```python
from build123d import *

# Parameters (mm, degrees)
BOSS_EXTRUDE1_DEPTH     = 106
SKETCH3_R               = 5
BOSS_EXTRUDE2_DEPTH     = 61.5
BOSS_EXTRUDE3_START     = -25
BOSS_EXTRUDE3_DEPTH     = 70.666666667
BOSS_EXTRUDE4_DEPTH     = 2.5
FILLET2_R               = 10
CUT_EXTRUDE1_DEPTH      = 107
CUT_EXTRUDE1_DEPTH_BACK = 26
SKETCH7_R               = 20
SKETCH7_R_2             = 10
BOSS_EXTRUDE5_DEPTH     = 106
CUT_EXTRUDE2_DEPTH      = 1
CUT_EXTRUDE2_DEPTH_BACK = 132


with BuildPart() as part:
    # Sketch2 → Boss-Extrude1 (new body)
    with BuildSketch(Plane(origin=(0, 0, 0), x_dir=(1, 0, 0), z_dir=(0, 1, 0))):
        Polygon((0, -61.5), (0, 61.5), (-106, 0), align=None)
        Polygon((-10, 44.136889641), (-86.073338243, 0), (-10, -44.136889641), align=None, mode=Mode.SUBTRACT)
    extrude(amount=BOSS_EXTRUDE1_DEPTH)

    # Sketch3 → Boss-Extrude2 (add, symmetric)
    with BuildSketch(Plane.XY):
        with BuildLine():
            Line((0, 0), (50, 0))
            Line((50, 0), (91.711375741, 35))
            Line((91.711375741, 35), (150.654022129, 35))
            Line((150.654022129, 35), (201, -25))
            Line((201, -25), (246, -25))
            Line((246, -25), (246, -19))
            Line((246, -19), (246, -5))
            Line((246, -5), (231, -5))
            ThreePointArc((231, -5), (223.928932188, -7.928932188), (221, -15))
            Line((221, -15), (221, -19))
            Line((221, -19), (203.797845949, -19))
            Line((203.797845949, -19), (153.451868078, 41))
            Line((153.451868078, 41), (89.527554335, 41))
            Line((89.527554335, 41), (47.816178594, 6))
            Line((47.816178594, 6), (0, 6))
            Line((0, 6), (0, 0))
        make_face()
        with Locations((231, -15)):
            Circle(SKETCH3_R, mode=Mode.SUBTRACT)
    extrude(amount=BOSS_EXTRUDE2_DEPTH, both=True)

    # Sketch4 → Boss-Extrude3 (add)
    with BuildSketch(Plane(origin=(0, 0, 0), x_dir=(1, 0, 0), z_dir=(0, 1, 0)).offset(BOSS_EXTRUDE3_START)):
        Polygon((246, -30), (246, 30), (291, 0), align=None)
        Polygon((256, 11.314829082), (272.972243623, 0), (256, -11.314829082), align=None, mode=Mode.SUBTRACT)
    extrude(amount=BOSS_EXTRUDE3_DEPTH)

    # Sketch5 → Boss-Extrude4 (add, symmetric)
    with BuildSketch(Plane.XY):
        with BuildLine():
            Line((0, 106), (183.326730095, 106))
            Line((183.326730095, 106), (233.952407843, 45.666666667))
            Line((233.952407843, 45.666666667), (246, 45.666666667))
            Line((246, 45.666666667), (246, -5))
            Line((246, -5), (231, -5))
            ThreePointArc((231, -5), (223.928932188, -7.928932188), (221, -15))
            Line((221, -15), (221, -19))
            Line((221, -19), (203.797845949, -19))
            Line((203.797845949, -19), (153.451868078, 41))
            Line((153.451868078, 41), (89.527554335, 41))
            Line((89.527554335, 41), (47.816178594, 6))
            Line((47.816178594, 6), (0, 6))
            Line((0, 6), (0, 106))
        make_face()
    extrude(amount=BOSS_EXTRUDE4_DEPTH, both=True)

    # Fillet2
    fillet2_edges = [part.edges().sort_by_distance(p)[0] for p in [
        (50, 0, 0),
        (91.711375741, 35, 0),
        (150.654022129, 35, 0),
        (201, -25, 0),
        (203.797845949, -19, 32),
        (153.451868078, 41, 32),
        (89.527554335, 41, 32),
        (47.816178594, 6, 32),
        (47.816178594, 6, -32),
        (89.527554335, 41, -32),
        (153.451868078, 41, -32),
        (203.797845949, -19, -32),
        (233.952407843, 45.666666667, 0),
        (183.326730095, 106, 0),
    ]]
    fillet(fillet2_edges, radius=FILLET2_R)

    # Sketch6 → Cut-Extrude1 (cut, two sides)
    with BuildSketch(Plane(origin=(0, 0, 0), x_dir=(1, 0, 0), z_dir=(0, 1, 0))) as cut_extrude1_sk:
        Polygon((0, 61.5), (246, 61.5), (246, 30), align=None)
        Polygon((0, -61.5), (246, -30), (246, -61.5), align=None)
    extrude(amount=CUT_EXTRUDE1_DEPTH, mode=Mode.SUBTRACT)
    extrude(cut_extrude1_sk.sketch, amount=-CUT_EXTRUDE1_DEPTH_BACK, mode=Mode.SUBTRACT)

    # Sketch7 → Boss-Extrude5 (add)
    with BuildSketch(Plane(origin=(0, 0, 0), x_dir=(1, 0, 0), z_dir=(0, 1, 0))):
        with Locations((-10, 0)):
            Circle(SKETCH7_R)
        with Locations((-10, 0)):
            Circle(SKETCH7_R_2, mode=Mode.SUBTRACT)
    extrude(amount=BOSS_EXTRUDE5_DEPTH)

    # Sketch8 → Cut-Extrude2 (cut, two sides)
    with BuildSketch(Plane(origin=(0, 106, 0), x_dir=(1, 0, 0), z_dir=(0, 1, 0))) as cut_extrude2_sk:
        with BuildLine():
            Line((-86.073338243, 0), (-10, 44.136889641))
            Line((-10, 44.136889641), (-10, 10))
            ThreePointArc((-10, 10), (0, 0), (-10, -10))
            Line((-10, -10), (-10, -44.136889641))
            Line((-10, -44.136889641), (-86.073338243, 0))
        make_face()
    extrude(amount=CUT_EXTRUDE2_DEPTH, mode=Mode.SUBTRACT)
    extrude(cut_extrude2_sk.sketch, amount=-CUT_EXTRUDE2_DEPTH_BACK, mode=Mode.SUBTRACT)


solid = part.part
```
CAD build for the part. Positions are in the model's coordinates, mm. A direction names the side the tool comes from. Round coordinates to 2 decimals unless told otherwise and drop trailing zeros. Order: outer loops, then holes, each group sorted by start corner. A loop starts at its lowest first (then second) coordinate and runs counter-clockwise, first axis right, second up. Notation, with made-up numbers: (-28.5, 69.5) -> (1.5, 69.5) arc R17 cw to (1.5, 81.5) -> close; hole circle Ø8 at (67, 35.25). An arc over 180 degrees is marked (long way). Write item = value, one per line.
(1) 3-axis set-ups, long thin cutter, end or side, ignore diameter. For faces 5 (the flat face through (68.92, 23.71, -28.39)), 6 (the cylindrical face through (152.96, 40.09, 22.19)), 7 (the flat face through (-10, 52, -27)): which of +Z, -Z, +X, -X, +Y, -Y reach the whole face in a straight line?
Answers follow:
face_5 = -Z, +Y
face_6 = +Z, +Y
face_7 = +Y, -Y
(2) Drill centre lines: L1, parallel to Y at x = 231, z = -9.5; L2, parallel to X at y = -15, z = 0; L3, parallel to X at y = -15, z = 3. Where is each one in solid material? Low to high.
Answers follow:
L1 = -25 to -20, -10 to -5
L2 = 192.61 to 226, 236 to 256, 272.97 to 291
L3 = 192.61 to 200.44, 221 to 226, 236 to 256, 268.47 to 286.5
(3) Cut at B-B (x = -19). Write the cut outline in (y, z).
Answers follow:
outline = (0, -50.48) -> (106, -50.48) -> (106, -38.92) -> (0, -38.92) -> close; (0, 38.92) -> (106, 38.92) -> (106, 50.48) -> (0, 50.48) -> close
(4) Flat gauge pins, fed straight in: P1, Ø1.2, axis at y = -16.5, z = -19, coming from the -X side; P2, Ø2, axis at y = -16, z = 20, coming from the -X side; P3, Ø2, axis at x = 90.5, y = 63, coming from the -Z side. Where does each tip first touch, or does it go through?
Answers follow:
P1 = 193.36
P2 = 192.61
P3 = -2.5
(5) Cut at A-A (y = 16.5). State how many separate pieces and enclosed holes the cut face has, plus the area to 3 significant figures.
Answers follow:
separate_pieces = 2
enclosed_holes = 2
area = 6,630 mm²
(6) Pull direction X, two halves, no side cores. Call faces 1 (the flat face through (160.02, 25.27, -41.01)), 2 (the flat face through (246, 20, 16)), 3 (the flat face through (3, 0, 1)), 4 (the flat face through (121, 41, -26)): +X half, -X half, draft (parallel to the pull), parting line (faces both ways), or undercut.
Answers follow:
face_1 = +X half
face_2 = undercut
face_3 = draft
face_4 = undercut
(7) Cut at C-C (y = 92). Write the cut outline in (x, z), plus the area to 3 significant figures.
Answers follow:
outline = (-106, 0) -> (0, -61.5) -> (0, -17.32) arc R20 ccw to (9.84, -2.5) -> (195.07, -2.5) -> (195.07, 2.5) -> (9.84, 2.5) arc R20 ccw to (0, 17.32) -> (0, 61.5) -> close; hole (-86.07, 0) -> (-10, -44.14) -> (-10, -10) arc R10 ccw to (-10, 10) -> (-10, 44.14) -> close
area = 4,180 mm²
(8) Cut at D-D (x = 116). Write the cut outline in (y, z).
Answers follow:
outline = (35, -46.65) -> (41, -46.65) -> (41, -2.5) -> (106, -2.5) -> (106, 2.5) -> (41, 2.5) -> (41, 46.65) -> (35, 46.65) -> close
